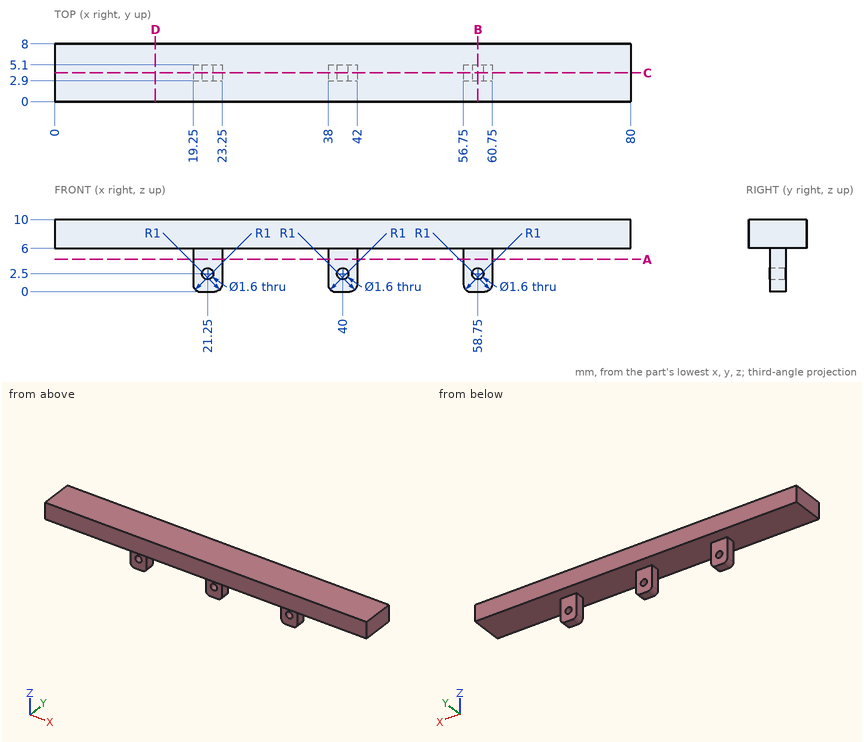
Job drawing, mm, ordinate dimensions from the low corner. One solid piece. Give positions to 0.01 mm unless a question says otherwise; leave off trailing zeros. Loops run counter-clockwise (first coordinate to the right, second up) from the corner with the lowest first, then second, coordinate; pieces in that order, holes last. Notation, with made-up numbers: M 16.25,69 L 49.25,69 A28 ccw 49.25,93 Z; hole C 38,22 d10. An arc over 180 degrees is marked long. Put each result on its own line as item: value. Start each with the question number.
1) Saw through at B-B (x = 58.75). List the corners of the cut face in (y, z), then the cut area to 3 significant figures.
2) Saw through at D-D (x = 14). List the corners of the cut face in (y, z).
3) Saw through at C-C (y = 4). List the corners of the cut face in (x, z).
4) Saw through at A-A (z = 4.5). List the corners of the cut face in (x, y), then the cut area to 3 significant figures.
5) Probe probe 1 along Z at (x, y) = (58.75, 4.6); probe 2 along Z at (x, y) = (41, 5.25). List the from-to ranges inside material, lowest first.
6) Flat gauge pins, fed straight in: pin 1 (1.2 mm diameter, centred on x = 21, z = 3.5, fed in from +Y); pin 2 (1.1 mm diameter, centred on y = 4, z = 4, fed in from +X); pin 3 (0.7 mm diameter, centred on y = 4, z = 4, fed in from -X); pin 4 (5 mm diameter, centred on x = 32, z = 2, fed in from -Y). Where does each tip first touch, or does it go through?
Numbers:
1. outline: M 0,6 L 2.9,6 L 2.9,3.3 L 5.1,3.3 L 5.1,6 L 8,6 L 8,10 L 0,10 Z; M 2.9,0 L 5.1,0 L 5.1,1.7 L 2.9,1.7 Z
1. area: 41.7 mm^2
2. outline: M 0,6 L 8,6 L 8,10 L 0,10 Z
3. outline: M 0,6 L 19.25,6 L 19.25,1 A1 ccw 20.25,0 L 22.25,0 A1 ccw 23.25,1 L 23.25,6 L 38,6 L 38,1 A1 ccw 39,0 L 41,0 A1 ccw 42,1 L 42,6 L 56.75,6 L 56.75,1 A1 ccw 57.75,0 L 59.75,0 A1 ccw 60.75,1 L 60.75,6 L 80,6 L 80,10 L 0,10 Z; hole C 21.25,2.5 d1.6; hole C 40,2.5 d1.6; hole C 58.75,2.5 d1.6
4. outline: M 19.25,2.9 L 23.25,2.9 L 23.25,5.1 L 19.25,5.1 Z; M 38,2.9 L 42,2.9 L 42,5.1 L 38,5.1 Z; M 56.75,2.9 L 60.75,2.9 L 60.75,5.1 L 56.75,5.1 Z
4. area: 26.4 mm^2
5. probe 1: 0 to 1.7, 3.3 to 10
5. probe 2: 6 to 10
6. pin 1: y = 5.1
6. pin 2: x = 60.75
6. pin 3: x = 19.25
6. pin 4: through
